```python
from build123d import *

# Parameters (mm, degrees)
F0_R     = 8.300329
F1_DEPTH = 52.6
F2_DEPTH = 6


with BuildPart() as f1:
    # F0 (on Top) → F1 (new body)
    with BuildSketch(Plane.XY):
        Circle(F0_R)
    extrude(amount=F1_DEPTH)

    # F0 (on Top) → F2 (join)
    with BuildSketch(Plane.XY):
        with BuildLine():
            ThreePointArc((17.74679, 13.770643), (17.113653, 14.549985), (16.44632, 15.300253))
            ThreePointArc((16.44632, 15.300253), (11.23142, 19.45339), (5.027248, 21.893057))
            ThreePointArc((5.027248, 21.893057), (4.04383, 22.095851), (3.052332, 22.254493))
            ThreePointArc((3.052332, 22.254493), (2.797639, 21.224553), (2.206503, 20.343529))
            ThreePointArc((2.206503, 20.343529), (10.23142, 17.721339), (16.514761, 12.082652))
            ThreePointArc((16.514761, 12.082652), (16.982183, 13.035103), (17.74679, 13.770643))
        make_face()
        with BuildLine():
            ThreePointArc((3.052332, 22.254493), (4.04383, 22.095851), (5.027248, 21.893057))
            ThreePointArc((5.027248, 21.893057), (0, 27.522274), (-5.027248, 21.893057))
            ThreePointArc((-5.027248, 21.893057), (-4.04383, 22.095851), (-3.052332, 22.254493))
            ThreePointArc((-3.052332, 22.254493), (-0.104234, 25.520498), (3.059434, 22.46284))
            ThreePointArc((3.059434, 22.46284), (3.057658, 22.358606), (3.052332, 22.254493))
        make_face()
        with BuildLine():
            ThreePointArc((20.799122, 8.48385), (21.157483, 7.545866), (21.473568, 6.592804))
            ThreePointArc((21.473568, 6.592804), (23.834989, 13.761137), (16.44632, 15.300253))
            ThreePointArc((16.44632, 15.300253), (17.113653, 14.549985), (17.74679, 13.770643))
            ThreePointArc((17.74679, 13.770643), (20.89195, 13.931547), (22.512824, 11.23142))
            ThreePointArc((22.512824, 11.23142), (22.049283, 9.612322), (20.799122, 8.48385))
        make_face()
        with BuildLine():
            ThreePointArc((21.473568, -6.592804), (22.214145, -3.333306), (22.46284, 0))
            ThreePointArc((22.46284, 0), (22.214145, 3.333306), (21.473568, 6.592804))
            ThreePointArc((21.473568, 6.592804), (21.157483, 7.545866), (20.799122, 8.48385))
            ThreePointArc((20.799122, 8.48385), (19.779822, 8.18945), (18.721265, 8.260876))
            ThreePointArc((18.721265, 8.260876), (20.022713, 4.221231), (20.46284, 0))
            ThreePointArc((20.46284, 0), (20.022713, -4.221231), (18.721265, -8.260876))
            ThreePointArc((18.721265, -8.260876), (19.779822, -8.18945), (20.799122, -8.48385))
            ThreePointArc((20.799122, -8.48385), (21.157483, -7.545866), (21.473568, -6.592804))
        make_face()
        with BuildLine():
            ThreePointArc((5.027248, -21.893057), (11.23142, -19.45339), (16.44632, -15.300253))
            ThreePointArc((16.44632, -15.300253), (17.113653, -14.549985), (17.74679, -13.770643))
            ThreePointArc((17.74679, -13.770643), (16.982183, -13.035103), (16.514761, -12.082652))
            ThreePointArc((16.514761, -12.082652), (10.23142, -17.721339), (2.206503, -20.343529))
            ThreePointArc((2.206503, -20.343529), (2.797639, -21.224553), (3.052332, -22.254493))
            ThreePointArc((3.052332, -22.254493), (4.04383, -22.095851), (5.027248, -21.893057))
        make_face()
        with BuildLine():
            ThreePointArc((16.44632, -15.300253), (23.834989, -13.761137), (21.473568, -6.592804))
            ThreePointArc((21.473568, -6.592804), (21.157483, -7.545866), (20.799122, -8.48385))
            ThreePointArc((20.799122, -8.48385), (22.049283, -9.612322), (22.512824, -11.23142))
            ThreePointArc((22.512824, -11.23142), (20.89195, -13.931547), (17.74679, -13.770643))
            ThreePointArc((17.74679, -13.770643), (17.113653, -14.549985), (16.44632, -15.300253))
        make_face()
        with BuildLine():
            ThreePointArc((-5.027248, -21.893057), (0, -27.522274), (5.027248, -21.893057))
            ThreePointArc((5.027248, -21.893057), (4.04383, -22.095851), (3.052332, -22.254493))
            ThreePointArc((3.052332, -22.254493), (3.057658, -22.358606), (3.059434, -22.46284))
            ThreePointArc((3.059434, -22.46284), (-0.104234, -25.520498), (-3.052332, -22.254493))
            ThreePointArc((-3.052332, -22.254493), (-4.04383, -22.095851), (-5.027248, -21.893057))
        make_face()
        with BuildLine():
            ThreePointArc((-16.44632, -15.300253), (-11.23142, -19.45339), (-5.027248, -21.893057))
            ThreePointArc((-5.027248, -21.893057), (-4.04383, -22.095851), (-3.052332, -22.254493))
            ThreePointArc((-3.052332, -22.254493), (-2.797639, -21.224553), (-2.206503, -20.343529))
            ThreePointArc((-2.206503, -20.343529), (-10.23142, -17.721339), (-16.514761, -12.082652))
            ThreePointArc((-16.514761, -12.082652), (-16.982183, -13.035103), (-17.74679, -13.770643))
            ThreePointArc((-17.74679, -13.770643), (-17.113653, -14.549985), (-16.44632, -15.300253))
        make_face()
        with BuildLine():
            ThreePointArc((-20.799122, 8.48385), (-21.157483, 7.545866), (-21.473568, 6.592804))
            ThreePointArc((-21.473568, 6.592804), (-22.46284, 0), (-21.473568, -6.592804))
            ThreePointArc((-21.473568, -6.592804), (-21.157483, -7.545866), (-20.799122, -8.48385))
            ThreePointArc((-20.799122, -8.48385), (-19.779822, -8.18945), (-18.721265, -8.260876))
            ThreePointArc((-18.721265, -8.260876), (-20.46284, 0), (-18.721265, 8.260876))
            ThreePointArc((-18.721265, 8.260876), (-19.779822, 8.18945), (-20.799122, 8.48385))
        make_face()
        with BuildLine():
            ThreePointArc((-3.052332, 22.254493), (-4.04383, 22.095851), (-5.027248, 21.893057))
            ThreePointArc((-5.027248, 21.893057), (-11.23142, 19.45339), (-16.44632, 15.300253))
            ThreePointArc((-16.44632, 15.300253), (-17.113653, 14.549985), (-17.74679, 13.770643))
            ThreePointArc((-17.74679, 13.770643), (-16.982183, 13.035103), (-16.514761, 12.082652))
            ThreePointArc((-16.514761, 12.082652), (-10.23142, 17.721339), (-2.206503, 20.343529))
            ThreePointArc((-2.206503, 20.343529), (-2.797639, 21.224553), (-3.052332, 22.254493))
        make_face()
        with BuildLine():
            ThreePointArc((-17.74679, 13.770643), (-17.113653, 14.549985), (-16.44632, 15.300253))
            ThreePointArc((-16.44632, 15.300253), (-23.834989, 13.761137), (-21.473568, 6.592804))
            ThreePointArc((-21.473568, 6.592804), (-21.157483, 7.545866), (-20.799122, 8.48385))
            ThreePointArc((-20.799122, 8.48385), (-22.102938, 12.761137), (-17.74679, 13.770643))
        make_face()
        with BuildLine():
            ThreePointArc((-21.473568, -6.592804), (-23.834989, -13.761137), (-16.44632, -15.300253))
            ThreePointArc((-16.44632, -15.300253), (-17.113653, -14.549985), (-17.74679, -13.770643))
            ThreePointArc((-17.74679, -13.770643), (-22.102938, -12.761137), (-20.799122, -8.48385))
            ThreePointArc((-20.799122, -8.48385), (-21.157483, -7.545866), (-21.473568, -6.592804))
        make_face()
        with BuildLine():
            ThreePointArc((20.46284, 0), (20.022713, 4.221231), (18.721265, 8.260876))
            ThreePointArc((18.721265, 8.260876), (16.803842, 9.701703), (16.514761, 12.082652))
            ThreePointArc((16.514761, 12.082652), (10.23142, 17.721339), (2.206503, 20.343529))
            ThreePointArc((2.206503, 20.343529), (0, 19.403406), (-2.206503, 20.343529))
            ThreePointArc((-2.206503, 20.343529), (-10.23142, 17.721339), (-16.514761, 12.082652))
            ThreePointArc((-16.514761, 12.082652), (-16.424308, 11.661301), (-16.393956, 11.23142))
            ThreePointArc((-16.393956, 11.23142), (-17.045068, 9.344591), (-18.721265, 8.260876))
            ThreePointArc((-18.721265, 8.260876), (-20.46284, 0), (-18.721265, -8.260876))
            ThreePointArc((-18.721265, -8.260876), (-17.045068, -9.344591), (-16.393956, -11.23142))
            ThreePointArc((-16.393956, -11.23142), (-16.424308, -11.661301), (-16.514761, -12.082652))
            ThreePointArc((-16.514761, -12.082652), (-10.23142, -17.721339), (-2.206503, -20.343529))
            ThreePointArc((-2.206503, -20.343529), (0, -19.403406), (2.206503, -20.343529))
            ThreePointArc((2.206503, -20.343529), (10.23142, -17.721339), (16.514761, -12.082652))
            ThreePointArc((16.514761, -12.082652), (16.803842, -9.701703), (18.721265, -8.260876))
            ThreePointArc((18.721265, -8.260876), (20.022713, -4.221231), (20.46284, 0))
        make_face()
        Circle(F0_R, mode=Mode.SUBTRACT)
    extrude(amount=F2_DEPTH)


solid = f1.part
```
Model file for the job. Use its own axes, mm. A direction names the side the tool comes from. Coordinates: 2 decimals unless noted, no trailing zeros. Write each loop counter-clockwise with the first axis right and the second up, starting at its lowest first coordinate (ties: lowest second). Pieces come first, ordered by that corner, then holes. Notation, with made-up numbers: (82, 24.25) - (101, 24.25) arc R24 cw to (101, 50.25) - close; hole circle Ø1 at (48.25, -14.75). An arc over 180 degrees is marked (long way). Use a Markdown table: item, result. Add a question column.
Item 1: 3-axis set-ups, long thin cutter, end or side, ignore diameter. For faces 1 (the face through (-23.89, -13.66, 2.96)), 2 (the face through (-6, 7, 6)): which of +Z, -Z, +X, -X, +Y, -Y reach the whole face in a straight line?
Item 2: Band-saw the part on B-B, the plane z = 18.5. Write the cut outline in (x, y).
Item 3: Band-saw the part on D-D, the plane x = -7. Write the cut outline in (y, z), and give its area (3 significant figures).
Item 4: Band-saw the part on C-C, the plane x = -20. Write the cut outline in (y, z), and give its area (3 significant figures).
Item 5: Two-plate mould, pull along Y, no slides. Class faces 3 (the face through (0, 0, 0)), 4 (the face through (23.89, 13.66, 2.96)), 5 (the face through (23.774, -13.864, 2.958)), 6 (the face through (7.92, 2.49, 28.97)): pulls with the +Y half, pulls with the -Y half, needs draft (parallel to the pull), parting line crosses it, or undercut.
Item 6: Drop flat-ended pins along their axis: pin 1 (12 mm diameter, centred on x = 6.5, z = 42, fed in from +Y); pin 2 (2 mm diameter, centred on x = -3.5, z = 14.5, fed in from -Y); pin 3 (6 mm diameter, centred on x = 5.5, z = 11.5, fed in from +Y). Give the stop position or say it passes through.
Item 7: Drill centre lines: line 1 along X through (y, z) = (-14, 2.5); line 2 along Z through (x, y) = (-14.5, -9); line 3 along Y through (x, z) = (0, 11.5). Where is each one in solid material? Low to high.
Item 8: Band-saw the part on A-A, the plane x = 0. Write the cut outline in (y, z), and give its area (3 significant figures).
A:
| question | item | result |
|---|---|---|
| 1 | face 1 | +Z, -Z |
| 1 | face 2 | +Z |
| 2 | outline | circle Ø16.6 at (0, 0) |
| 3 | outline | (-21.34, 0) - (21.34, 0) - (21.34, 6) - (4.46, 6) - (4.46, 52.6) - (-4.46, 52.6) - (-4.46, 6) - (-21.34, 6) - close |
| 3 | area | 672 mm² |
| 4 | outline | (-16.26, 0) - (-14.24, 0) - (-14.24, 6) - (-16.26, 6) - close; (-8.22, 0) - (8.22, 0) - (8.22, 6) - (-8.22, 6) - close; (14.24, 0) - (16.26, 0) - (16.26, 6) - (14.24, 6) - close |
| 4 | area | 123 mm² |
| 5 | face 3 | needs draft |
| 5 | face 4 | undercut |
| 5 | face 5 | undercut |
| 5 | face 6 | parting line crosses it |
| 6 | pin 1 | stops at y = 8.29 |
| 6 | pin 2 | stops at y = -7.91 |
| 6 | pin 3 | stops at y = 7.91 |
| 7 | line 1 | x = -23.69 to -20.76, -18.15 to 18.15, 20.76 to 23.69 |
| 7 | line 2 | z = 0 to 6 |
| 7 | line 3 | y = -8.3 to 8.3 |
| 8 | outline | (-27.52, 0) - (-25.52, 0) - (-25.52, 6) - (-27.52, 6) - close; (-19.4, 0) - (19.4, 0) - (19.4, 6) - (8.3, 6) - (8.3, 52.6) - (-8.3, 52.6) - (-8.3, 6) - (-19.4, 6) - close; (25.52, 0) - (27.52, 0) - (27.52, 6) - (25.52, 6) - close |
| 8 | area | 1,030 mm² |
